For this review, take the finished solid that the model builds, in its own axes (mm). A direction names the side the tool comes from. Coordinates: 2 decimals unless noted, no trailing zeros. Write each loop counter-clockwise with the first axis right and the second up, starting at its lowest first coordinate (ties: lowest second). Pieces come first, ordered by that corner, then holes. Notation, with made-up numbers: M 18.5,22 L 76.5,22 A16 cw 76.5,33 Z; hole C 42,-9 d7. An arc over 180 degrees is marked long. One line per question, with ' | ' between items.
from build123d import *

# Parameters (mm, degrees)
BOSS_EXTRUDE1_DEPTH = 10
BOSS_EXTRUDE2_START = 1
BOSS_EXTRUDE2_DEPTH = 1
SKETCH3_R           = 4
BOSS_EXTRUDE3_DEPTH = 6
SKETCH4_R           = 3
BOSS_EXTRUDE4_DEPTH = 15
FILLET1_R           = 2


with BuildPart() as part:
    # Sketch1 → Boss-Extrude1 (new body)
    with BuildSketch(Plane(origin=(0, 0, 0), x_dir=(1, 0, 0), z_dir=(0, 1, 0))):
        with BuildLine():
            Line((-20.000157194, 1.500878546), (-20.000157194, -1.500878546))
            Line((-20.000157194, -1.500878546), (-0.880639137, -4.921836518))
            ThreePointArc((-0.880639137, -4.921836518), (0, -5), (0.880639137, -4.921836518))
            Line((0.880639137, -4.921836518), (20.000157194, -1.500878546))
            Line((20.000157194, -1.500878546), (20.000157194, 1.500878546))
            Line((20.000157194, 1.500878546), (0.880639137, 4.921836518))
            ThreePointArc((0.880639137, 4.921836518), (0, 5), (-0.880639137, 4.921836518))
            Line((-0.880639137, 4.921836518), (-20.000157194, 1.500878546))
        make_face()
        with BuildLine():
            Line((-19.000157194, -0.663922493), (-19.000157194, 0.663922493))
            Line((-19.000157194, 0.663922493), (-18.824029366, 0.695436148))
            Line((-18.824029366, 0.695436148), (-3.65761322, 3.409085733))
            ThreePointArc((-3.65761322, 3.409085733), (-5, 0), (-3.65761322, -3.409085733))
            Line((-3.65761322, -3.409085733), (-18.824029366, -0.695436148))
            Line((-18.824029366, -0.695436148), (-19.000157194, -0.663922493))
        make_face(mode=Mode.SUBTRACT)
        with BuildLine():
            Line((18.824029366, 0.695436148), (19.000157194, 0.663922493))
            Line((19.000157194, 0.663922493), (19.000157194, -0.663922493))
            Line((19.000157194, -0.663922493), (18.824029366, -0.695436148))
            Line((18.824029366, -0.695436148), (3.65761322, -3.409085733))
            ThreePointArc((3.65761322, -3.409085733), (5, 0), (3.65761322, 3.409085733))
            Line((3.65761322, 3.409085733), (18.824029366, 0.695436148))
        make_face(mode=Mode.SUBTRACT)
    extrude(amount=BOSS_EXTRUDE1_DEPTH)

    # Sketch2 → Boss-Extrude2 (add)
    with BuildSketch(Plane.XZ.offset(BOSS_EXTRUDE2_START)):
        with BuildLine():
            Line((-20.000157194, 1.500878546), (-0.880639137, 4.921836518))
            ThreePointArc((-0.880639137, 4.921836518), (0, 5), (0.880639137, 4.921836518))
            Line((0.880639137, 4.921836518), (20.000157194, 1.500878546))
            Line((20.000157194, 1.500878546), (20.000157194, -1.500878546))
            Line((20.000157194, -1.500878546), (0.880639137, -4.921836518))
            ThreePointArc((0.880639137, -4.921836518), (0, -5), (-0.880639137, -4.921836518))
            Line((-0.880639137, -4.921836518), (-20.000157194, -1.500878546))
            Line((-20.000157194, -1.500878546), (-20.000157194, 1.500878546))
        make_face()
    extrude(amount=-BOSS_EXTRUDE2_DEPTH)

    # Sketch3 → Boss-Extrude3 (add)
    with BuildSketch(Plane(origin=(0, 10, 0), x_dir=(1, 0, 0), z_dir=(0, 1, 0))):
        with Locations(Location((0, 0, 0), (0, 0, 270))):
            Circle(SKETCH3_R)
    extrude(amount=BOSS_EXTRUDE3_DEPTH)

    # Sketch4 → Boss-Extrude4 (add)
    with BuildSketch(Plane(origin=(0, 16, 0), x_dir=(1, 0, 0), z_dir=(0, 1, 0))):
        with Locations(Location((0, 0, 0), (0, 0, 270))):
            Circle(SKETCH4_R)
    extrude(amount=BOSS_EXTRUDE4_DEPTH)

    # Fillet1
    # the kernel refuses this fillet: 2 mm, written as the material it takes off along each edge
    with BuildSketch(Plane(origin=(20.000157194, -5.184780263, 1.500878546), x_dir=(-0.9843673036221247, 0, 0.17612782732920945), z_dir=(0, 1, 0)), Plane(origin=(20.000157194, -5.184780263, -1.500878546), x_dir=(0, 0, 1), z_dir=(0, 1, 0)), Plane(origin=(-20.000157194, 14.184780263, 1.500878546), x_dir=(0.9843673036221245, 0, 0.17612782732920956), z_dir=(0, -1, 0))) as fillet1_piece_1:
        with BuildLine():
            CenterArc((FILLET1_R * 0.836956052521, -FILLET1_R), FILLET1_R, 90, 79.855702636)
            Line((-FILLET1_R * 0.147411251101, -FILLET1_R * 0.823872172671), (0, 0))
            Line((0, 0), (FILLET1_R * 0.836956052521, 0))
        make_face()
    extrude(amount=19.369560525, mode=Mode.SUBTRACT)
    with BuildSketch(Plane(origin=(-20.000157194, -5.184780263, -1.500878546), x_dir=(0, 0, 1), z_dir=(0, 1, 0))) as fillet1_piece_2:
        with BuildLine():
            CenterArc((FILLET1_R * 0.836956052521, FILLET1_R), FILLET1_R, 190.144297364, 79.855702636)
            Line((-FILLET1_R * 0.147411251101, FILLET1_R * 0.823872172671), (0, 0))
            Line((0, 0), (FILLET1_R * 0.836956052521, 0))
        make_face()
    extrude(amount=19.369560525, mode=Mode.SUBTRACT)


solid = part.part
1. Take a section at D-D on z = -1.25. State the section outline as (x, y) points.
Computed values:
outline: M -19.41,-1 L 19.41,-1 L 19.41,10 L 15.72,10 L 15.72,0 L 4.84,0 L 4.84,10 L 3.8,10 L 3.8,16 L 2.73,16 L 2.73,31 L -2.73,31 L -2.73,16 L -3.8,16 L -3.8,10 L -4.84,10 L -4.84,0 L -15.72,0 L -15.72,10 L -19.41,10 Z
2. Draft analysis for pull direction Z (two halves, no side actions). For faces 3 (the cylindrical face through (-3.905, 12.958, -0.867)), 4 (the flat face through (-11, 0, 0)), 5 (the cylindrical face through (19.49, 4.42, -1.16)), 6 (the cylindrical face through (-19.464, 4.577, 1.189)), state which applies: pulls with the +Z half, pulls with the -Z half, needs draft (parallel to the pull), parting line crosses it, or undercut.
Computed values:
face 3: parting line crosses it | face 4: undercut | face 5: pulls with the -Z half | face 6: pulls with the +Z half
3. Take a section at C-C on y = 19. State the section outline as (x, z) points, plus the area to 3 significant figures.
Computed values:
outline: C 0,0 d6 | area: 28.3 mm2
4. For line 1 along X through (y, z) = (1, 0.5); line 2 along Y through (x, z) = (12, 2.25); line 3 along Z through (x, y) = (-12.5, 7.5), list the stretches that pass through material, from the lowest coordinate up.
Computed values:
line 1: x = -19.88 to -19, -4.97 to 4.97, 19 to 19.88 | line 2: y = -1 to 10 | line 3: z = -2.84 to -1.83, 1.83 to 2.84
5. Take a section at A-A on x = 0. State the section outline as (y, z) points, plus the area to 3 significant figures.
Computed values:
outline: M -1,-5 L 10,-5 L 10,-4 L 16,-4 L 16,-3 L 31,-3 L 31,3 L 16,3 L 16,4 L 10,4 L 10,5 L -1,5 Z | area: 248 mm2
6. Machinability: for faces 1 (the cylindrical face through (0, 4, -5)), 2 (the cylindrical face through (0.9, 23.4, 2.86)), which of the approach directions +Z, -Z, +X, -X, +Y, -Y give a long, thin tool a straight path to every point of the face, cutting with its end or side? Answer none if there is none.
Computed values:
face 1: -Z, +Y, -Y | face 2: +Y
7. Take a section at B-B on y = 8. State the section outline as (x, z) points.
Computed values:
outline: M -19.99,0 A2 ccw -18.35,-1.8 L -0.88,-4.92 A5 ccw 0.88,-4.92 L 18.35,-1.8 A2 ccw 19.99,0 A2 ccw 18.35,1.8 L 0.88,4.92 A5 ccw -0.88,4.92 L -18.35,1.8 A2 ccw Z; hole M -19,-0.66 L -3.66,-3.41 A5 cw -3.66,3.41 L -19,0.66 Z; hole M 3.66,-3.41 L 19,-0.66 L 19,0.66 L 3.66,3.41 A5 cw Z
8. Clearance check with flat-ended pins moving along their axes: P1, Ø2, axis at x = 12.5, z = 0, coming from the +Y side; P2, Ø5, axis at x = 6, y = 14, coming from the -Z side; P3, Ø5, axis at y = 11.5, z = 2, coming from the -X side; P4, Ø1, axis at x = 12, y = 8.5, coming from the -Z side. State where each tip first meets the part, or that it passes through.
Computed values:
P1: stops at y = 0 | P2: stops at z = -1.94 | P3: stops at x = -19.99 | P4: stops at z = -3.02
